from build123d import *

# Parameters (mm, degrees)
F0_W     = 304.8
F0_H     = 304.8
F1_DEPTH = 6.35
F3_D     = 6.6
F4_D     = 8.8


with BuildPart() as f1:
    # F0 (on Top) → F1 (new body)
    with BuildSketch(Plane.XY):
        Rectangle(F0_W, F0_H)
    extrude(amount=F1_DEPTH)

    # F3 (through all)
    with Locations(Plane.XY.offset(6.35)):
        with Locations((-81.35, -110), (-66.35, -95), (-81.35, -80), (-81.35, 80), (-66.35, 95), (-81.35, 110), (114.75, 39.7726856172), (114.75, -39.7726856172)):
            Hole(F3_D / 2)

    # F4 (through all)
    with Locations(Plane.XY.offset(6.35)):
        with Locations((114.75, 0)):
            Hole(F4_D / 2)


solid = f1.part
Model file for the job. Use its own axes, mm. Coordinates: 2 decimals unless noted, no trailing zeros. Return JSON: item names as keys, results as strings. Group by question number.
Item 1: Flat gauge pin, fed straight in: P1, Ø5.5, axis at x = -81.35, y = -80, coming from the -Z side. Where does the tip first touch, or does it go through?
Item 2: Pull direction X, two halves, no side cores. Call faces 1 (the cylindrical face through (-83.1, 82.8, 3.1)), 2 (the flat face through (-2, 2, 0)): pulls with the +X half, pulls with the -X half, needs draft (parallel to the pull), parting line crosses it, or undercut.
Item 3: Wall check: line 1 along Y through (x, z) = (114.75, 5.25); line 2 along Y through (x, z) = (-81.35, 3.5); line 3 along Y through (x, z) = (-66.35, 3). Give the ranges that are in metal, low to high. Write a range as [from, to].
Values found:
{
 "1": {"P1": "passes through"},
 "2": {"face 1": "undercut", "face 2": "needs draft"},
 "3": {"line 1": "y = [-152.4, -43.07], [-36.47, -4.4], [4.4, 36.47], [43.07, 152.4]", "line 2": "y = [-152.4, -113.3], [-106.7, -83.3], [-76.7, 76.7], [83.3, 106.7], [113.3, 152.4]", "line 3": "y = [-152.4, -98.3], [-91.7, 91.7], [98.3, 152.4]"}
}
